Design review of the part built by this model. Coordinates are the model's own, in mm. A direction names the side the tool comes from. Coordinates: 2 decimals unless noted, no trailing zeros. Write each loop counter-clockwise with the first axis right and the second up, starting at its lowest first coordinate (ties: lowest second). Pieces come first, ordered by that corner, then holes. Notation, with made-up numbers: M 37,-17 L 70,-17 A27 cw 70,5 Z; hole C -5.5,86.25 d7. An arc over 180 degrees is marked long. One line per question, with ' | ' between items.
from build123d import *

# Parameters (mm, degrees)
SKETCH1_R           = 9
BOSS_EXTRUDE1_DEPTH = 65
SKETCH2_R           = 6.576456623
SKETCH2_R_2         = 5.146719103
CUT_EXTRUDE2_DEPTH  = 1
FILLET1_R           = 1
CHAMFER1_SIZE       = 1
SKETCH3_R           = 8.24633038
SKETCH3_R_2         = 7.786680871
CUT_EXTRUDE3_DEPTH  = 0.4
FILLET2_R           = 0.1


with BuildPart() as part:
    # Sketch1 → Boss-Extrude1 (new body)
    with BuildSketch(Plane.XY):
        Circle(SKETCH1_R)
    extrude(amount=BOSS_EXTRUDE1_DEPTH)

    # Sketch2 → Cut-Extrude2 (cut)
    with BuildSketch(Plane.XY.offset(65)):
        Circle(SKETCH2_R)
        Circle(SKETCH2_R_2, mode=Mode.SUBTRACT)
    extrude(amount=-CUT_EXTRUDE2_DEPTH, mode=Mode.SUBTRACT)

    # Fillet1
    fillet1_edges = [part.edges().sort_by_distance(p)[0] for p in [
        (-9, 0, 65),
    ]]
    fillet(fillet1_edges, radius=FILLET1_R)

    # Chamfer1
    chamfer1_edges = [part.edges().sort_by_distance(p)[0] for p in [
        (-5.146719103, 0, 65),
    ]]
    chamfer(chamfer1_edges, length=CHAMFER1_SIZE - 0.0001)  # a hair under: the kernel refuses the full size

    # Sketch3 → Cut-Extrude3 (cut)
    with BuildSketch(Plane(origin=(0, 0, 0), x_dir=(-1, 0, 0), z_dir=(0, 0, -1))):
        Circle(SKETCH3_R)
        Circle(SKETCH3_R_2, mode=Mode.SUBTRACT)
    extrude(amount=-CUT_EXTRUDE3_DEPTH, mode=Mode.SUBTRACT)

    # Fillet2
    fillet2_edges = [part.edges().sort_by_distance(p)[0] for p in [
        (-9, 0, 0),
    ]]
    fillet(fillet2_edges, radius=FILLET2_R)


solid = part.part
1. Tool access review of faces 1 (the face through (0, 0, 0)), 2 (the face through (6.54, -5.02, 0.2)), 3 (the face through (-5, -2, 64)): name each direction out of +Z, -Z, +X, -X, +Y, -Y from which nothing blocks a thin tool from reaching the whole face with its end or side.
Answer sheet:
face 1: -Z, +X, -X, +Y, -Y | face 2: -Z | face 3: +Z
2. Insertion check: pin 1 Ø1 at (y, z) = (3.5, 50.5) entering from +X; pin 2 Ø8 at (x, z) = (-7, 35.5) entering from +Y; pin 3 Ø2 at (y, z) = (6, 25.5) entering from -X. Each pin has a flat end and moves straight along its axis. Give the tip position at first contact, or say it passes through.
Answer sheet:
pin 1: x = 8.49 | pin 2: y = 8.49 | pin 3: x = -7.48
3. Take a section at A-A (z = 6). Write out the cut boundary in (x, y).
Answer sheet:
outline: C 0,0 d18
4. Draft analysis for pull direction X (two halves, no side actions). For faces 4 (the face through (-1.172, 8.923, 31.603)), 5 (the face through (3, -8, 0)), 6 (the face through (-1.43, -6.42, 64.51)), state which applies: pulls with the +X half, pulls with the -X half, needs draft (parallel to the pull), parting line crosses it, or undercut.
Answer sheet:
face 4: parting line crosses it | face 5: needs draft | face 6: undercut
5. To check wall thickness, follow line 1 along Y through (x, z) = (0, 0.2); line 2 along Y through (x, z) = (0, 64.2); line 3 along X through (y, z) = (-4.5, 28). State the ranges of each line that lie inside material, in increasing order. Write a range as [from, to].
Answer sheet:
line 1: [-9, -8.25], [-7.79, 7.79], [8.25, 9] | line 2: [-8.98, -6.58], [-4.95, 4.95], [6.58, 8.98] | line 3: [-7.79, 7.79]
